Source: CAD feature listing. Evaluate the final solid. Frame: model axes, mm. Face numbers are marked on the shaded views. A direction names the side the tool comes from. Give positions to 0.01 mm unless a question says otherwise; leave off trailing zeros. Order: outer loops, then holes, each group sorted by start corner. A loop starts at its lowest first (then second) coordinate and runs counter-clockwise, first axis right, second up. Notation, with made-up numbers: M 61,35 L 76,35 A18 cw 76,53 Z; hole C 46,-17 d8. An arc over 180 degrees is marked long. Answer as a JSON object with one key per item and string values. Group by question number.
1. Set-up query: the marked faces 5, 6 and 7. Return all of +Z, -Z, +X, -X, +Y, -Y with unobstructed straight access to the full face (end or side cutting, diameter ignored); none if empty.
2. Section query B-B (z = 16). Output: boundary loops of the cut face in (x, y), plus the area to 3 significant figures.
3. Material intervals for L1, parallel to Z at x = -17.5, y = 1.7; L2, parallel to Z at x = 2, y = 0.4; L3, parallel to X at y = 0.75, z = -1, sorted ascending. Write a range as [from, to].
4. Pull-direction query (X, two-part tool) for the marked faces 1, 2, 3 and 4; classes: +X half, -X half, draft (parallel to the pull), parting line (faces both ways), or undercut.
5. Pin query (flat end, axial travel): P1, Ø12, axis at x = -2, z = 6.5, coming from the -Y side; P2, Ø3, axis at x = -7, y = 2, coming from the -Z side; P3, Ø3, axis at y = 1, z = 9.5, coming from the +X side. Return the tip coordinate at first contact, or that it passes through.
6. Section query A-A (x = -9). Output: boundary loops of the cut face in (y, z).
from build123d import *

# Parameters (mm, degrees)
BOSS_EXTRUDE1_DEPTH = 5
FILLET1_R           = 2


with BuildPart() as part:
    # Sketch1 → Boss-Extrude1 (new body)
    with BuildSketch(Plane(origin=(0, 0, 0), x_dir=(1, 0, 0), z_dir=(0, 1, 0))):
        with BuildLine():
            Line((5.177710586, -20.063712518), (2.831257578, -9.590827937))
            ThreePointArc((2.831257578, -9.590827937), (7.071067812, -7.071067812), (9.590827937, -2.831257578))
            Line((9.590827937, -2.831257578), (20.063712518, -5.177710586))
            Line((20.063712518, -5.177710586), (20.063712518, 0.338076022))
            Line((20.063712518, 0.338076022), (19.877881915, 5.850731362))
            Line((19.877881915, 5.850731362), (9.489996307, 3.152771812))
            ThreePointArc((9.489996307, 3.152771812), (7.071067812, 7.071067812), (3.152771812, 9.489996307))
            Line((3.152771812, 9.489996307), (5.850731362, 19.877881915))
            Line((5.850731362, 19.877881915), (0.338076022, 20.063712518))
            Line((0.338076022, 20.063712518), (-5.177710586, 20.063712518))
            Line((-5.177710586, 20.063712518), (-2.831257578, 9.590827937))
            ThreePointArc((-2.831257578, 9.590827937), (-7.071067812, 7.071067812), (-9.590827937, 2.831257578))
            Line((-9.590827937, 2.831257578), (-20.063712518, 5.177710586))
            Line((-20.063712518, 5.177710586), (-20.063712518, -0.338076022))
            Line((-20.063712518, -0.338076022), (-19.877881915, -5.850731362))
            Line((-19.877881915, -5.850731362), (-9.489996307, -3.152771812))
            ThreePointArc((-9.489996307, -3.152771812), (-7.071067812, -7.071067812), (-3.152771812, -9.489996307))
            Line((-3.152771812, -9.489996307), (-5.850731362, -19.877881915))
            Line((-5.850731362, -19.877881915), (-0.338076022, -20.063712518))
            Line((-0.338076022, -20.063712518), (5.177710586, -20.063712518))
        make_face()
        Polygon((-0.338076022, -0.721880139), (-0.338076022, -0.338076022), (-0.721880139, -0.338076022), (-0.721880139, 0.338076022), (-0.338076022, 0.338076022), (-0.338076022, 0.721880139), (0.012163769, 0.721880139), (0.362204732, 0.710080322), (0.34927411, 0.326494088), (0.732860345, 0.313563466), (0.722290178, 0), (0.732860345, -0.313563466), (0.34927411, -0.326494088), (0.362204732, -0.710080322), (0.012163769, -0.721880139), align=None, mode=Mode.SUBTRACT)
    extrude(amount=BOSS_EXTRUDE1_DEPTH)

    # Fillet1
    fillet1_edges = [part.edges().sort_by_distance(p)[0] for p in [
        (20.063712518, 2.5, 5.177710586),
        (-5.850731362, 2.5, 19.877881915),
        (-20.063712518, 2.5, -5.177710586),
        (5.850731362, 2.5, -19.877881915),
    ]]
    fillet(fillet1_edges, radius=FILLET1_R)


solid = part.part
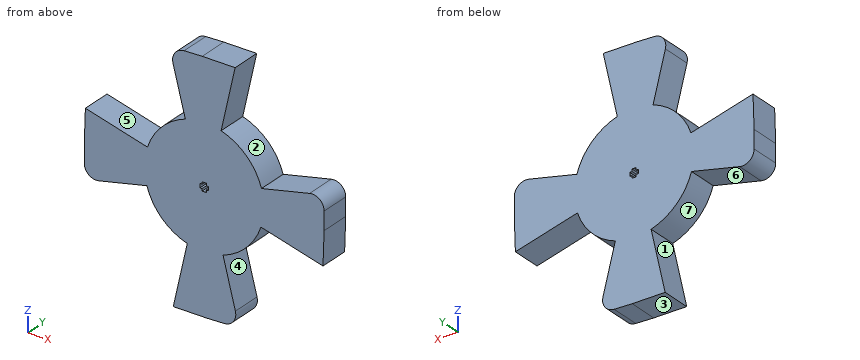
Answer sheet:
{
 "1": {"face 5": "+Z, +Y, -Y", "face 6": "-Z, +Y, -Y", "face 7": "+Y, -Y"},
 "2": {"outline": "M -4.84,0 L 4.27,0 L 4.27,5 L -4.84,5 Z", "area": "45.6 mm^2"},
 "3": {"L1": "[-4.6, 5.23]", "L2": "[-20.01, 20.06]", "L3": "[-20.06, 20.04]"},
 "4": {"face 1": "-X half", "face 2": "undercut", "face 3": "draft", "face 4": "+X half"},
 "5": {"P1": "y = 0", "P2": "z = -8.35", "P3": "x = 6"},
 "6": {"outline": "M 0,-4.36 L 5,-4.36 L 5,4.36 L 0,4.36 Z"}
}
